Job drawing, mm, ordinate dimensions from the low corner. One solid piece. A direction names the side the tool comes from. Round coordinates to 2 decimals unless told otherwise and drop trailing zeros. Loops run counter-clockwise (first coordinate to the right, second up) from the corner with the lowest first, then second, coordinate; pieces in that order, holes last.
1) Band-saw the part on C-C, the plane y = 1.75. Write the cut outline in (x, z), then the cut area to 3 significant figures.
2) 3-axis set-ups, long thin cutter, end or side, ignore diameter. For the marked faces 1, 2, 3 and 4: which of +Z, -Z, +X, -X, +Y, -Y reach the whole face in a straight line?
3) Drop a flat-ended pin along its axis: P1, Ø4, axis at y = 3.5, z = 25, coming from the +X side. Give the stop position or say it passes through.
4) Band-saw the part on B-B, the plane x = 43.75. State how many separate pieces and enclosed holes the cut face has, then the cut area to 3 significant figures.
5) Probe line 1 (X direction, y = 5, z = 33.75); line 2 (Z direction, x = 48, y = 5). List the from-to ranges inside material, lowest first.
6) Band-saw the part on A-A, the plane z = 9. Write the cut outline in (x, y).
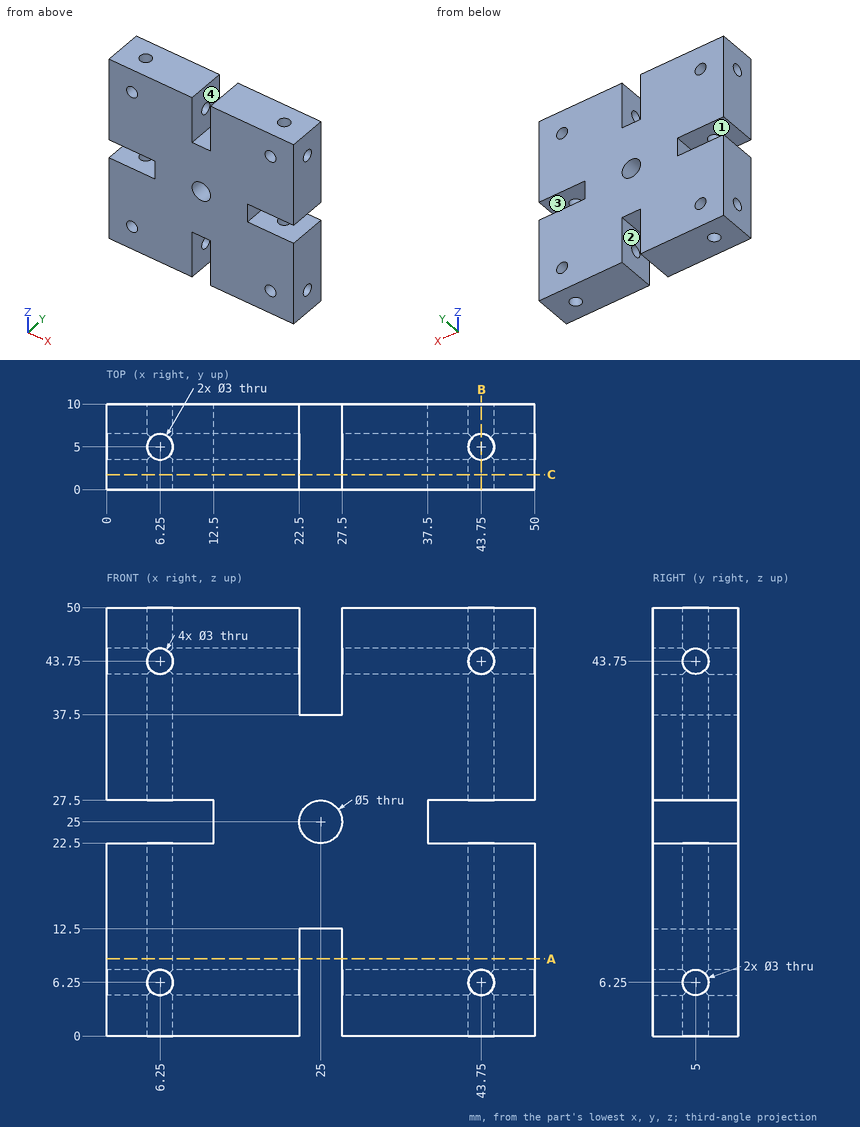
Reported:
1. outline: (0, 0) - (22.5, 0) - (22.5, 12.5) - (27.5, 12.5) - (27.5, 0) - (50, 0) - (50, 22.5) - (37.5, 22.5) - (37.5, 27.5) - (50, 27.5) - (50, 50) - (27.5, 50) - (27.5, 37.5) - (22.5, 37.5) - (22.5, 50) - (0, 50) - (0, 27.5) - (12.5, 27.5) - (12.5, 22.5) - (0, 22.5) - close; hole circle Ø3 at (6.25, 6.25); hole circle Ø3 at (6.25, 43.75); hole circle Ø5 at (25, 25); hole circle Ø3 at (43.75, 6.25); hole circle Ø3 at (43.75, 43.75)
1. area: 2,200 mm2
2. face 1: -X, +Y, -Y
2. face 2: -Z, +Y, -Y
2. face 3: +X, +Y, -Y
2. face 4: +Z, +Y, -Y
3. P1: stops at x = 37.5
4. separate pieces: 8
4. enclosed holes: 0
4. area: 273 mm2
5. line 1: x = 0 to 4.75, 7.75 to 42.25, 45.25 to 50
5. line 2: z = 0 to 4.75, 7.75 to 22.5, 27.5 to 42.25, 45.25 to 50
6. outline: (0, 0) - (22.5, 0) - (22.5, 10) - (0, 10) - close; (27.5, 0) - (50, 0) - (50, 10) - (27.5, 10) - close; hole circle Ø3 at (6.25, 5); hole circle Ø3 at (43.75, 5)
